The listing builds one solid part. Answer for the finished solid, in the listing's coordinates (mm). A direction names the side the tool comes from. Give positions to 0.01 mm unless a question says otherwise; leave off trailing zeros. Loops run counter-clockwise (first coordinate to the right, second up) from the corner with the lowest first, then second, coordinate; pieces in that order, holes last. Notation, with made-up numbers: M 46.25,62.25 L 70.25,62.25 A9 ccw 70.25,78.25 Z; hole C 1,18.25 d7. An arc over 180 degrees is marked long. One line per item, written item: value. Start each with the question number.
Q1. Flat-ended cylindrical pins translate along their axes: pin 1 (1.4 mm diameter, centred on x = 1, z = 0.5, fed in from +Y); pin 2 (1 mm diameter, centred on x = -4.5, z = 5, fed in from +Y). Find the tip coordinate at first contact, or state that the pin passes through.
Q2. Consider L1, parallel to Z at x = -4.3, y = -9.3; L2, parallel to Z at x = -0.2, y = -1.75; L3, parallel to X at y = -1, z = -5.5. Determine where each line is inside the solid, lowest interval first.
Q3. The mould has two halves that part along Z. Classify faces 1 (the flat face through (4, -11.2, -4)), 2 (the flat face through (0, -5, -8)), 3 (the flat face through (4, -9.6, -4)): +Z half, -Z half, draft (parallel to the pull), parting line (faces both ways), or undercut.
Q4. A cutting plane is placed at C-C, the plane z = -4.4. Determine the outline of the cut face in (x, y), and give its area (3 significant figures).
Q5. A cutting plane is placed at A-A, the plane y = -6.25. Determine the outline of the cut face in (x, z), and give its area (3 significant figures).
Q6. A cutting plane is placed at B-B, the plane x = 4.3. Determine the outline of the cut face in (y, z), and give its area (3 significant figures).
Q7. A cutting plane is placed at D-D, the plane x = -0.2. Determine the outline of the cut face in (y, z), and give its area (3 significant figures).
Q8. For faces 4 (the flat face through (-4, -11.2, 4)), 5 (the flat face through (1, -8.1, -3)), 6 (the cylindrical face through (2.6, -10.39, -2.85)), determine the directions among +Z, -Z, +X, -X, +Y, -Y from which every point of the face is accessible in a straight line to the end or side of a thin tool.
from build123d import *

# Parameters (mm, degrees)
F0_W     = 16
F0_H     = 16
F0_W_2   = 12.8
F0_H_2   = 12.8
F1_DEPTH = 9.6
F2_DEPTH = 8.1
F3_R     = 1.6
F4_DEPTH = 1.6
F5_R     = 2.3
F6_DEPTH = 1.6
F7_R     = 3.2
F7_R_2   = 2.4
F8_DEPTH = 9.6


with BuildPart() as f1:
    # F0 (on Front) → F1 (new body)
    with BuildSketch(Plane.XZ):
        Rectangle(F0_W, F0_H)
        Rectangle(F0_W_2, F0_H_2, mode=Mode.SUBTRACT)
        Rectangle(F0_W_2, F0_H_2)
    extrude(amount=F1_DEPTH)

    # F0 (on Front) → F2 (cut)
    with BuildSketch(Plane.XZ):
        Rectangle(F0_W_2, F0_H_2)
    extrude(amount=F2_DEPTH, mode=Mode.SUBTRACT)

    # F3 (on face) → F4 (cut)
    with BuildSketch(Plane.XZ.offset(9.6)):
        with Locations((-4.3, 4.4)):
            Circle(F3_R)
        with Locations((-4.3, -4.4)):
            Circle(F3_R)
        with Locations((4.3, 4.4)):
            Circle(F3_R)
        with Locations((4.3, -4.4)):
            Circle(F3_R)
    extrude(amount=-F4_DEPTH, mode=Mode.SUBTRACT)

    # F5 (on face) → F6 (join)
    with BuildSketch(Plane.XZ.offset(9.6)):
        with Locations((-4.3, 4.4)):
            Circle(F5_R)
        with Locations((-4.3, -4.4)):
            Circle(F5_R)
        with Locations((4.3, 4.4)):
            Circle(F5_R)
        with Locations((4.3, -4.4)):
            Circle(F5_R)
    extrude(amount=F6_DEPTH)

    # F7 (on face) → F8 (join)
    with BuildSketch(Plane.XZ.offset(9.6)):
        with Locations((-0.2, 0.2)):
            Circle(F7_R)
        with Locations((-0.2, 0.2)):
            Circle(F7_R_2, mode=Mode.SUBTRACT)
    extrude(amount=-F8_DEPTH)


solid = f1.part
Answer block:
1. pin 1: y = -8.1
1. pin 2: y = -9.6
2. L1: -8 to -6, -2.8 to 2.8, 6 to 8
2. L2: -8 to -6.4, -3 to -2.2, 2.6 to 3.4, 6.4 to 8
2. L3: -8 to -6.4, 6.4 to 8
3. face 1: draft
3. face 2: -Z half
3. face 3: undercut
4. outline: M -8,-9.6 L -6.6,-9.6 L -6.6,-11.2 L -2,-11.2 L -2,-9.6 L 2,-9.6 L 2,-11.2 L 6.6,-11.2 L 6.6,-9.6 L 8,-9.6 L 8,0 L 6.4,0 L 6.4,-8.1 L 5.9,-8.1 L 5.9,-9.6 L 2.7,-9.6 L 2.7,-8.1 L -2.7,-8.1 L -2.7,-9.6 L -5.9,-9.6 L -5.9,-8.1 L -6.4,-8.1 L -6.4,0 L -8,0 Z
4. area: 55.0 mm^2
5. outline: M -8,-8 L 8,-8 L 8,8 L -8,8 Z; C -0.2,0.2 d6.4; hole M -6.4,-6.4 L 6.4,-6.4 L 6.4,6.4 L -6.4,6.4 Z; hole C -0.2,0.2 d4.8
5. area: 106 mm^2
6. outline: M -11.2,-6.7 L -9.6,-6.7 L -9.6,-8 L 0,-8 L 0,-6.4 L -8.1,-6.4 L -8.1,-6 L -9.6,-6 L -9.6,-2.8 L -8.1,-2.8 L -8.1,2.8 L -9.6,2.8 L -9.6,6 L -8.1,6 L -8.1,6.4 L 0,6.4 L 0,8 L -9.6,8 L -9.6,6.7 L -11.2,6.7 L -11.2,2.1 L -9.6,2.1 L -9.6,-2.1 L -11.2,-2.1 Z
6. area: 55.0 mm^2
7. outline: M -9.6,-8 L 0,-8 L 0,-6.4 L -8.1,-6.4 L -8.1,-3 L 0,-3 L 0,-2.2 L -8.1,-2.2 L -8.1,2.6 L 0,2.6 L 0,3.4 L -8.1,3.4 L -8.1,6.4 L 0,6.4 L 0,8 L -9.6,8 Z
7. area: 62.9 mm^2
8. face 4: +Z, -Z, +X, -X, -Y
8. face 5: +Y
8. face 6: -Y
